```python
from build123d import *

# Parameters (mm, degrees)
SKETCH1_W           = 5.3
SKETCH1_H           = 5.3
BOSS_EXTRUDE1_DEPTH = 5
SKETCH2_R           = 3.95
BOSS_EXTRUDE2_DEPTH = 7
SKETCH3_R           = 1.95
BOSS_EXTRUDE3_DEPTH = 11
CUT_EXTRUDE1_DEPTH  = 11


with BuildPart() as part:
    # Sketch1 → Boss-Extrude1 (new body)
    with BuildSketch(Plane(origin=(0, 0, 0), x_dir=(1, 0, 0), z_dir=(0, 1, 0))):
        with Locations((0, 0.143071786)):
            Rectangle(SKETCH1_W, SKETCH1_H)
    extrude(amount=BOSS_EXTRUDE1_DEPTH)

    # Sketch2 → Boss-Extrude2 (add)
    with BuildSketch(Plane(origin=(0, 5, 0), x_dir=(1, 0, 0), z_dir=(0, 1, 0))):
        Circle(SKETCH2_R)
    extrude(amount=BOSS_EXTRUDE2_DEPTH)

    # Sketch3 → Boss-Extrude3 (add)
    with BuildSketch(Plane(origin=(0, 12, 0), x_dir=(1, 0, 0), z_dir=(0, 1, 0))):
        Circle(SKETCH3_R)
    extrude(amount=BOSS_EXTRUDE3_DEPTH)

    # Sketch4 → Cut-Extrude1 (cut)
    with BuildSketch(Plane(origin=(0, 23, 0), x_dir=(1, 0, 0), z_dir=(0, 1, 0))):
        with BuildLine():
            Line((-1.754992877, 0.85), (1.754992877, 0.85))
            ThreePointArc((1.754992877, 0.85), (0, 1.95), (-1.754992877, 0.85))
        make_face()
    extrude(amount=-CUT_EXTRUDE1_DEPTH, mode=Mode.SUBTRACT)


solid = part.part
```
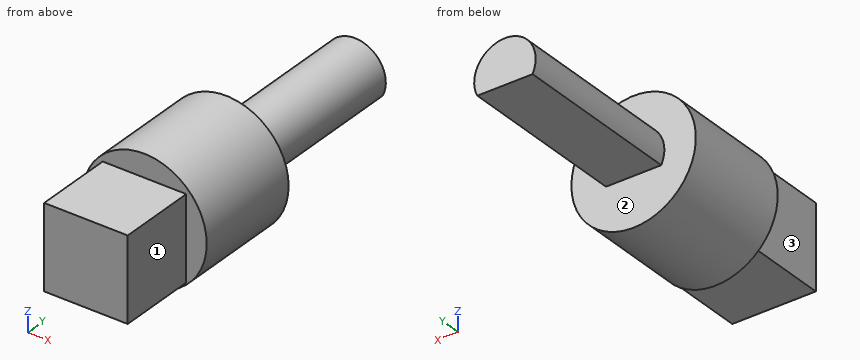
Geometry: final body of the model. Coordinates: model frame, mm. Face numbers are marked on the shaded views. A direction names the side the tool comes from. Coordinates: 2 decimals unless noted, no trailing zeros. Order: outer loops, then holes, each group sorted by start corner. A loop starts at its lowest first (then second) coordinate and runs counter-clockwise, first axis right, second up. Notation, with made-up numbers: (42.25, 84.5) - (60.25, 84.5) arc R22 ccw to (60.25, 108.5) - close; hole circle Ø11 at (50, 41). An arc over 180 degrees is marked (long way). Return JSON: item names as keys, results as strings. Group by question number.
1. Pin query (flat end, axial travel): pin 1 (1 mm diameter, centred on y = 4, z = 0, fed in from +X); pin 2 (4 mm diameter, centred on x = -2, y = 12, fed in from +Z); pin 3 (1.5 mm diameter, centred on x = 0.5, y = 3, fed in from +Z); pin 4 (1 mm diameter, centred on x = -0.5, z = -2.5, fed in from +Y). Return the tip coordinate at first contact, or that it passes through.
2. Cut plane C-C (y = 11.5). Output: boundary loops of the cut face in (x, z).
3. Cut plane B-B (x = 0). Output: boundary loops of the cut face in (y, z).
4. Cut plane D-D (y = 14.75). Output: boundary loops of the cut face in (x, z) (3 decimals), plus the area to 3 significant figures.
5. Set-up query: the marked faces 1, 2 and 3. Return all of +Z, -Z, +X, -X, +Y, -Y with unobstructed straight access to the full face (end or side cutting, diameter ignored); none if empty.
6. Cut plane A-A (z = 0). Output: boundary loops of the cut face in (x, y).
7. Material intervals for line 1 along Z through (x, y) = (0.5, 2.5); line 2 along Y through (x, z) = (0, 2); line 3 along Y through (x, z) = (2.75, -2), sorted ascending. Write a range as [from, to].
Resolved:
{
 "1": {"pin 1": "stops at x = 2.65", "pin 2": "stops at z = 3.95", "pin 3": "stops at z = 2.51", "pin 4": "stops at y = 12"},
 "2": {"outline": "circle Ø7.9 at (0, 0)"},
 "3": {"outline": "(0, -2.79) - (5, -2.79) - (5, -3.95) - (12, -3.95) - (12, -0.85) - (23, -0.85) - (23, 1.95) - (12, 1.95) - (12, 3.95) - (5, 3.95) - (5, 2.51) - (0, 2.51) - close"},
 "4": {"outline": "(-1.755, -0.85) - (1.755, -0.85) arc R1.95 ccw (long way) to start", "area": "9.18 mm²"},
 "5": {"face 1": "+Z, -Z, +X, -Y", "face 2": "+Y", "face 3": "+Z, -Z, -X, -Y"},
 "6": {"outline": "(-3.95, 5) - (-2.65, 5) - (-2.65, 0) - (2.65, 0) - (2.65, 5) - (3.95, 5) - (3.95, 12) - (1.95, 12) - (1.95, 23) - (-1.95, 23) - (-1.95, 12) - (-3.95, 12) - close"},
 "7": {"line 1": "z = [-2.79, 2.51]", "line 2": "y = [0, 12]", "line 3": "y = [5, 12]"}
}
